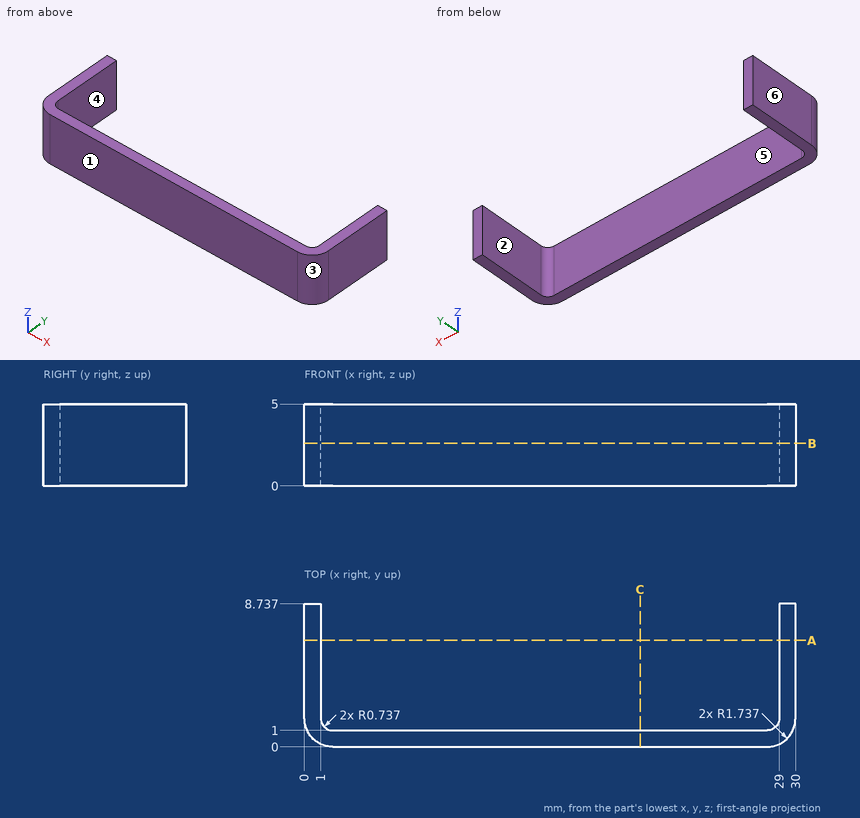
The drawing under review shows one solid part. Ordinate dimensions are in mm from its lowest x, y, z. A direction names the side the tool comes from. Coordinates: 2 decimals unless noted, no trailing zeros. Write each loop counter-clockwise with the first axis right and the second up, starting at its lowest first coordinate (ties: lowest second). Pieces come first, ordered by that corner, then holes. Notation, with made-up numbers: (38.5, 62) -> (76.5, 62) arc R27 ccw to (76.5, 100) -> close; hole circle Ø1 at (45.5, 43.25). An arc over 180 degrees is marked (long way). Write each question's results on one line, items separated by ' | '. Start each with the question number.
1) For the marked faces 5 and 6, list the 3-axis set-ups (+Z, -Z, +X, -X, +Y, -Y) from which the entire face can be reached by the end or side of a thin tool; tool diameter is ignored.
2) Insertion check: pin 1 (2.5 mm diameter, centred on x = 17, z = 2, fed in from +Y); pin 2 (2.5 mm diameter, centred on y = 4, z = 3, fed in from -X). Each pin has a flat end and moves straight along its axis. Give the tip position at first contact, or say it passes through.
3) Wall thickness on L1, parallel to X at y = 5.75, z = 1; L2, parallel to Y at x = 27, z = 2.35: over which ranges is each line inside the solid? List them lowest first. Write a range as [from, to].
4) The part is to be moulded in two halves that separate along X. For the marked faces 1, 2, 3 and 4, say which applies: +X half, -X half, draft (parallel to the pull), parting line (faces both ways), or undercut.
5) Consider section C-C (x = 20.5). Write out the cut boundary in (y, z).
6) Consider section B-B (z = 2.6). Write out the cut boundary in (x, y).
7) Consider section A-A (y = 6.5). Write out the cut boundary in (x, z).
Geometry says:
1) face 5: +Z, -Z, +Y | face 6: +Z, -Z, -X, +Y, -Y
2) pin 1: y = 1 | pin 2: x = 0
3) L1: [0, 1], [29, 30] | L2: [0, 1]
4) face 1: draft | face 2: undercut | face 3: +X half | face 4: undercut
5) outline: (0, 0) -> (1, 0) -> (1, 5) -> (0, 5) -> close
6) outline: (0, 1.74) arc R1.74 ccw to (1.74, 0) -> (28.26, 0) arc R1.74 ccw to (30, 1.74) -> (30, 8.74) -> (29, 8.74) -> (29, 1.74) arc R0.74 cw to (28.26, 1) -> (1.74, 1) arc R0.74 cw to (1, 1.74) -> (1, 8.74) -> (0, 8.74) -> close
7) outline: (0, 0) -> (1, 0) -> (1, 5) -> (0, 5) -> close; (29, 0) -> (30, 0) -> (30, 5) -> (29, 5) -> close
